CAD build for the part. Positions are in the model's coordinates, mm. Face numbers are marked on the shaded views. A direction names the side the tool comes from. Round coordinates to 2 decimals unless told otherwise and drop trailing zeros. Order: outer loops, then holes, each group sorted by start corner. A loop starts at its lowest first (then second) coordinate and runs counter-clockwise, first axis right, second up. Notation, with made-up numbers: M 64,65.5 L 93,65.5 A28 cw 93,95.5 Z; hole C -19,62.25 d8. An arc over 180 degrees is marked long. Put each result on its own line as item: value.
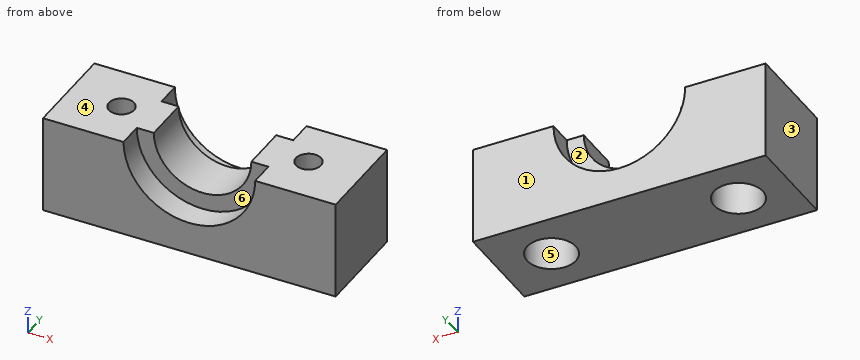
```python
from build123d import *

# Parameters (mm, degrees)
F0_W     = 36
F0_H     = 12
F0_R     = 3
F0_R_2   = 1.55
F1_DEPTH = 12.09
F2_DEPTH = 10
F4_DEPTH = 12
F5_DEPTH = 3.1
F7_DEPTH = 3.1


with BuildPart() as f1:
    # F0 (on Top) → F1 (new body)
    with BuildSketch(Plane.XY):
        Rectangle(F0_W, F0_H)
        with Locations((-11.5, 0)):
            Circle(F0_R, mode=Mode.SUBTRACT)
        with Locations((11.5, 0)):
            Circle(F0_R, mode=Mode.SUBTRACT)
        with Locations((11.5, 0)):
            Circle(F0_R)
        with Locations((11.5, 0)):
            Circle(F0_R_2, mode=Mode.SUBTRACT)
        with Locations((-11.5, 0)):
            Circle(F0_R)
        with Locations((-11.5, 0)):
            Circle(F0_R_2, mode=Mode.SUBTRACT)
    extrude(amount=F1_DEPTH)

    # F0 (on Top) → F2 (cut)
    with BuildSketch(Plane.XY):
        with Locations((-11.5, 0)):
            Circle(F0_R)
        with Locations((-11.5, 0)):
            Circle(F0_R_2, mode=Mode.SUBTRACT)
        with Locations((11.5, 0)):
            Circle(F0_R)
        with Locations((11.5, 0)):
            Circle(F0_R_2, mode=Mode.SUBTRACT)
    extrude(amount=F2_DEPTH, mode=Mode.SUBTRACT)

    # F3 (on face) → F4 (cut, through all)
    with BuildSketch(Plane.XZ.offset(6)):
        with BuildLine():
            Line((6, 12.09), (-6, 12.09))
            ThreePointArc((-6, 12.09), (0, 6.09), (6, 12.09))
        make_face()
    extrude(amount=-F4_DEPTH, mode=Mode.SUBTRACT)

    # F3 (on face) → F5 (cut)
    with BuildSketch(Plane.XZ.offset(6)):
        with BuildLine():
            Line((-6, 12.09), (-8.1, 12.09))
            ThreePointArc((-8.1, 12.09), (0, 3.99), (8.1, 12.09))
            Line((8.1, 12.09), (6, 12.09))
            ThreePointArc((6, 12.09), (0, 6.09), (-6, 12.09))
        make_face()
    extrude(amount=-F5_DEPTH, mode=Mode.SUBTRACT)

    # F6 (on face) → F7 (cut)
    with BuildSketch(Plane(origin=(0, 6, 0), x_dir=(-1, 0, 0), z_dir=(0, 1, 0))):
        with BuildLine():
            Line((-6, 12.09), (-8.1, 12.09))
            ThreePointArc((-8.1, 12.09), (0, 3.99), (8.1, 12.09))
            Line((8.1, 12.09), (6, 12.09))
            ThreePointArc((6, 12.09), (0, 6.09), (-6, 12.09))
        make_face()
    extrude(amount=-F7_DEPTH, mode=Mode.SUBTRACT)


solid = f1.part
```
Item 1: Probe line 1 along X through (y, z) = (0.5, 10.5); line 2 along X through (y, z) = (-1, 1.75); line 3 along Y through (x, z) = (-11.5, 10.8). List the from-to ranges inside material, lowest first. Write a range as [from, to].
Answers below:
line 1: [-18, -12.97], [-10.03, -5.79], [5.79, 10.03], [12.97, 18]
line 2: [-18, -14.33], [-8.67, 8.67], [14.33, 18]
line 3: [-6, -1.55], [1.55, 6]
Item 2: Band-saw the part on D-D on x = 0. Give the cut face in (y, z), and give its area (3 significant figures).
Answers below:
outline: M -6,0 L 6,0 L 6,3.99 L 2.9,3.99 L 2.9,6.09 L -2.9,6.09 L -2.9,3.99 L -6,3.99 Z
area: 60.1 mm²
Item 3: Band-saw the part on C-C on y = -4. Give the cut face in (x, z), and give its area (3 significant figures).
Answers below:
outline: M -18,0 L 18,0 L 18,12.09 L 8.1,12.09 A8.1 cw -8.1,12.09 L -18,12.09 Z
area: 332 mm²
Item 4: Band-saw the part on B-B on x = -11.5. Give the cut face in (y, z), and give its area (3 significant figures).
Answers below:
outline: M -6,0 L -3,0 L -3,10 L -1.55,10 L -1.55,12.09 L -6,12.09 Z; M 1.55,10 L 3,10 L 3,0 L 6,0 L 6,12.09 L 1.55,12.09 Z
area: 78.6 mm²
Item 5: Band-saw the part on A-A on z = 6.5. Give the cut face in (x, y).
Answers below:
outline: M -18,-6 L -5.86,-6 L -5.86,-2.9 L -2.18,-2.9 L -2.18,2.9 L -5.86,2.9 L -5.86,6 L -18,6 Z; M 2.18,-2.9 L 5.86,-2.9 L 5.86,-6 L 18,-6 L 18,6 L 5.86,6 L 5.86,2.9 L 2.18,2.9 Z; hole C -11.5,0 d6; hole C 11.5,0 d6
Item 6: Mould opens along X. For the marked faces 1, 2 and 3 say: pulls with the +X half, pulls with the -X half, needs draft (parallel to the pull), parting line crosses it, or undercut.
Answers below:
face 1: needs draft
face 2: undercut
face 3: pulls with the -X half
Item 7: Pin check, flat tips, straight feed: P1, Ø4, axis at x = 11.5, y = 0, coming from the +Z side; P2, Ø5.5, axis at x = -11.5, y = 0, coming from the -Z side; P3, Ø2.5, axis at x = -1.5, z = 8.5, coming from the +Y side. Stop position of each tip, or through.
Answers below:
P1: z = 12.09
P2: z = 10
P3: through
Item 8: Tool access for the marked faces 4, 5 and 6: list every direction of +Z, -Z, +X, -X, +Y, -Y with a clear straight run to the whole face (end or side of a thin tool).
Answers below:
face 4: +Z, +X, -X, +Y, -Y
face 5: -Z
face 6: +Z, -Y
